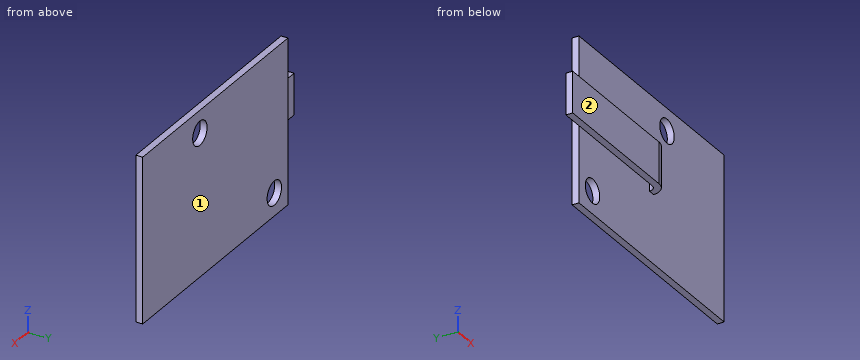
from build123d import *

# Parameters (mm, degrees)
SKETCH1_W                  = 35.3
SKETCH1_H                  = 24
BOSS_EXTRUDE1_DEPTH        = 1
F_3_5_3_5_DIAMETER_HOLE1_D = 3.5
SKETCH5_W                  = 1
SKETCH5_H                  = 6
BOSS_EXTRUDE2_DEPTH        = 2
SKETCH6_W                  = 6
SKETCH6_H                  = 1
BOSS_EXTRUDE3_DEPTH        = 22
FILLET1_R                  = 1
FILLET2_R                  = 2


with BuildPart() as part:
    # Sketch1 → Boss-Extrude1 (new body)
    with BuildSketch(Plane(origin=(0, 0, 0), x_dir=(1, 0, 0), z_dir=(0, 1, 0))):
        Rectangle(SKETCH1_W, SKETCH1_H)
    extrude(amount=BOSS_EXTRUDE1_DEPTH)

    # Ø3.5 (3.5) Diameter Hole1 (through all)
    with Locations(Plane(origin=(0, 1, 0), x_dir=(1, 0, 0), z_dir=(0, 1, 0))):
        with Locations((-14.35, 8.7), (3.75, -8.7)):
            Hole(F_3_5_3_5_DIAMETER_HOLE1_D / 2)

    # Sketch5 → Boss-Extrude2 (add)
    with BuildSketch(Plane.XZ):
        with Locations((0, 1)):
            Rectangle(SKETCH5_W, SKETCH5_H)
    extrude(amount=BOSS_EXTRUDE2_DEPTH)

    # Sketch6 → Boss-Extrude3 (add)
    with BuildSketch(Plane.ZY.offset(0.5)):
        with Locations((1, -1.5)):
            Rectangle(SKETCH6_W, SKETCH6_H)
    extrude(amount=BOSS_EXTRUDE3_DEPTH)

    # Fillet1
    fillet1_edges = [part.edges().sort_by_distance(p)[0] for p in [
        (-0.5, -1, 1),
    ]]
    fillet(fillet1_edges, radius=FILLET1_R - 0.0001)  # a hair under: the kernel refuses the full size

    # Fillet2
    fillet2_edges = [part.edges().sort_by_distance(p)[0] for p in [
        (0.5, -2, 1),
    ]]
    fillet(fillet2_edges, radius=FILLET2_R - 0.0001)  # a hair under: the kernel refuses the full size


solid = part.part
Read the model definition and answer for the solid it produces. Units are mm, in the model's axes. Face numbers are marked on the shaded views. Round coordinates to 2 decimals unless told otherwise and drop trailing zeros. Loops run counter-clockwise (first coordinate to the right, second up) from the corner with the lowest first, then second, coordinate; pieces in that order, holes last. Notation, with made-up numbers: (4, 29.5) - (43, 29.5) arc R23 cw to (43, 44.5) - close; hole circle Ø1 at (-17, -27). An arc over 180 degrees is marked (long way). One line per question, with ' | ' between items. Start each with the question number.
Q1. Section B-B on x = 3.75 is taken. Give the vertices of the cut face in (y, z), plus the area to 3 significant figures.
Q2. Flat-ended cylindrical pins translate along their axes: pin 1 (1 mm diameter, centred on x = -4.5, y = -1, fed in from +Z); pin 2 (1 mm diameter, centred on x = -7, y = -1.5, fed in from -Z); pin 3 (0.8 mm diameter, centred on y = 0.5, z = 2.5, fed in from -X). Find the tip coordinate at first contact, or state that the pin passes through.
Q3. Find the intervals of material crossed by L1, parallel to X at y = 0.7, z = 8.7; L2, parallel to Y at x = -9, z = -1; L3, parallel to Z at x = 3.75, y = 0.55, in increasing order.
Q4. Section A-A on z = -8.7 is taken. Give the vertices of the cut face in (x, y), plus the area to 3 significant figures.
Q5. Section D-D on z = -5 is taken. Give the vertices of the cut face in (x, y), plus the area to 3 significant figures.
Q6. For a pull along Y with two mould halves and no side action, classify the marked faces 1 and 2 as +Y half, -Y half, draft (parallel to the pull), parting line (faces both ways), or undercut.
Q7. Section C-C on x = -14.35 is taken. Give the vertices of the cut face in (y, z), plus the area to 3 significant figures.
Established:
1) outline: (0, -12) - (1, -12) - (1, 6.95) - (0, 6.95) - close; (0, 10.45) - (1, 10.45) - (1, 12) - (0, 12) - close | area: 20.5 mm²
2) pin 1: z = 4 | pin 2: z = -2 | pin 3: x = -17.65
3) L1: -17.65 to 2, 5.5 to 17.65 | L2: -2 to -1, 0 to 1 | L3: -12 to 6.95, 10.45 to 12
4) outline: (-17.65, 0) - (-16.1, 0) - (-16.1, 1) - (-17.65, 1) - close; (-12.6, 0) - (17.65, 0) - (17.65, 1) - (-12.6, 1) - close | area: 31.8 mm²
5) outline: (-17.65, 0) - (17.65, 0) - (17.65, 1) - (-17.65, 1) - close | area: 35.3 mm²
6) face 1: +Y half | face 2: -Y half
7) outline: (-2, -2) - (-1, -2) - (-1, 4) - (-2, 4) - close; (0, -12) - (1, -12) - (1, -10.45) - (0, -10.45) - close; (0, -6.95) - (1, -6.95) - (1, 12) - (0, 12) - close | area: 26.5 mm²
